from build123d import *

# Parameters (mm, degrees)
SKETCH_3_R               = 1.25
CUT_EXTRUDE_1_DEPTH      = 18.300578025
CHAMFER_1_SIZE           = 0.4
PATTERN_CIRCULAR_1_COUNT = 3


with BuildPart() as part:
    # Эскиз2 → Повернуть1 (revolve)
    with BuildSketch(Plane.XY, mode=Mode.PRIVATE) as revolve_1_sk:
        Polygon((0, 0), (0, 9.5), (-3.6, 9.5), (-3.6, 3.5), (-14.5, 3.5), (-14.5, 0), align=None)
    revolve(revolve_1_sk.sketch.rotate(Axis((-14.5, 0, 0), (1, 0, 0)), 90), axis=Axis((-14.5, 0, 0), (1, 0, 0)))

    # Эскиз3 → Вырез-Вытянуть1 (cut, through all)
    with BuildSketch(Plane.ZY.offset(3.6)):
        with Locations((0, 4.75)):
            Circle(SKETCH_3_R)
    cut_extrude_1 = extrude(amount=-CUT_EXTRUDE_1_DEPTH, mode=Mode.SUBTRACT)

    # Фаска1
    chamfer_1_edges = [part.edges().sort_by_distance(p)[0] for p in [
        (-14.5, 0, -3.5),
        (-3.6, 0, -9.5),
        (0, 0, -9.5),
    ]]
    chamfer(chamfer_1_edges, length=CHAMFER_1_SIZE)

    # Круговой массив1: Вырез-Вытянуть1 ×3 about axis
    pattern_circular_1_axis = Axis((0, 0, 0), (1, 0, 0))
    for i in range(1, PATTERN_CIRCULAR_1_COUNT):
        add(cut_extrude_1.rotate(pattern_circular_1_axis, i * 360 / PATTERN_CIRCULAR_1_COUNT), mode=Mode.SUBTRACT)


solid = part.part
The listing builds one solid part. Answer for the finished solid, in the listing's coordinates (mm). A direction names the side the tool comes from. Round coordinates to 2 decimals unless told otherwise and drop trailing zeros. Write each loop counter-clockwise with the first axis right and the second up, starting at its lowest first coordinate (ties: lowest second). Pieces come first, ordered by that corner, then holes. Notation, with made-up numbers: (59, 62) - (100, 62) arc R14 ccw to (100, 69) - close; hole circle Ø11 at (26.25, 18.5). An arc over 180 degrees is marked (long way). Use a Markdown table: item, result. Add a question column.
1. Consider line 1 (Y direction, x = -1.7, z = 0); line 2 (X direction, y = 6, z = 6.25); line 3 (Y direction, x = -6.25, z = 0). Determine where each line is inside the solid, lowest interval first.
2. The part is cut by section C-C (y = -2.25). Give the number of separate pieces and of enclosed holes in the cut face, and give its area (3 significant figures).
3. For a pull along Z with two mould halves and no side action, classify faces 3 (the face through (-1.825, -3.136, 3.122)), 4 (the face through (0, 0, 0)), 5 (the face through (-1.82, 9.274, -2.059)) as +Z half, -Z half, draft (parallel to the pull), parting line (faces both ways), or undercut.
4. The part is cut by section B-B (x = -8.5). Write down the section's boundary in (y, z), and give its area (3 significant figures).
5. Flat-ended cylindrical pins translate along their axes: P1, Ø6, axis at y = 0.5, z = 7, coming from the -X side; P2, Ø2, axis at y = 4.75, z = 0, coming from the +X side; P3, Ø2, axis at x = -3.5, z = -2, coming from the -Y side; P4, Ø2, axis at x = -6.5, y = -4, coming from the +Z side. Find the tip coordinate at first contact, or state that the pin passes through.
6. A tool of negligible diameter and unlimited length cuts with its end or side. For faces 1 (the face through (-1.83, 3.53, -0.27)), 2 (the face through (-3.6, 0, 4)), from which of +Z, -Z, +X, -X, +Y, -Y can it reach the whole face along a straight path? Write none if from no direction.
7. The part is cut by section A-A (y = 0). Write down the section's boundary in (x, z), and give its area (3 significant figures).
Reported:
| question | item | result |
|---|---|---|
| 1 | line 1 | -9.5 to 3.5, 6 to 9.5 |
| 1 | line 2 | -3.6 to 0 |
| 1 | line 3 | -3.5 to 3.5 |
| 2 | separate pieces | 3 |
| 2 | enclosed holes | 0 |
| 2 | area | 106 mm^2 |
| 3 | face 3 | undercut |
| 3 | face 4 | draft |
| 3 | face 5 | parting line |
| 4 | outline | circle Ø7 at (0, 0) |
| 4 | area | 38.5 mm^2 |
| 5 | P1 | x = -3.6 |
| 5 | P2 | through |
| 5 | P3 | y = -9.44 |
| 5 | P4 | z = 1.8 |
| 6 | face 1 | +X, -X |
| 6 | face 2 | -X |
| 7 | outline | (-14.5, -3.1) - (-14.1, -3.5) - (-3.6, -3.5) - (-3.6, -9.1) - (-3.2, -9.5) - (-0.4, -9.5) - (0, -9.1) - (0, 9.1) - (-0.4, 9.5) - (-3.2, 9.5) - (-3.6, 9.1) - (-3.6, 3.5) - (-14.1, 3.5) - (-14.5, 3.1) - close |
| 7 | area | 144 mm^2 |
